from build123d import *

# Parameters (mm, degrees)
F1_DEPTH = 112.7125


with BuildPart() as f1:
    # F0 (on Right) → F1 (new body, symmetric)
    with BuildSketch(Plane.YZ):
        with BuildLine():
            ThreePointArc((-65.019769, 11.612246), (-46.032427, -7.846355), (-24.695704, -24.695704))
            Line((-24.695704, -24.695704), (0, 0))
            Line((0, 0), (0, 34.925))
            ThreePointArc((0, 34.925), (-27.001631, 38.098052), (-54.187018, 37.764821))
            ThreePointArc((-54.187018, 37.764821), (-67.631541, 28.013901), (-65.019769, 11.612246))
        make_face()
    extrude(amount=F1_DEPTH, both=True)


solid = f1.part
The listing builds one solid part. Answer for the finished solid, in the listing's coordinates (mm). Round coordinates to 2 decimals unless told otherwise and drop trailing zeros. Loops run counter-clockwise (first coordinate to the right, second up) from the corner with the lowest first, then second, coordinate; pieces in that order, holes last. Notation, with made-up numbers: M 28,37 L 45,37 A12 cw 45,55 Z; hole C -8,66.5 d3. An arc over 180 degrees is marked long. Write each question's results on one line, items separated by ' | '. Start each with the question number.
1) Find section C-C on y = -12. Write down the section's boundary in (x, z).
2) Find section B-B on z = 28. Write down the section's boundary in (x, y).
3) Each of these flat-tipped pins is pushed along its axis until it touches: pin 1 (6 mm diameter, centred on x = -14, y = -14, fed in from +Z); pin 2 (8 mm diameter, centred on x = 22, y = -7, fed in from -Z); pin 3 (6 mm diameter, centred on x = 43, y = -12, fed in from +Z). Where does it stop, or does it pass through?
4) Find section A-A on x = 78. Write down the section's boundary in (y, z) (3 decimals).
5) Straight lines are drawn through the part: probe 1 along Y at (x, z) = (-83.5, 22.5); probe 2 along Z at (x, y) = (-90, -56); probe 3 along Y at (x, z) = (-39, -2.5). For each, find the intervals that lie inside material, in ascending order.
Final values:
1) outline: M -112.71,-12 L 112.71,-12 L 112.71,36.77 L -112.71,36.77 Z
2) outline: M -112.71,-67.64 L 112.71,-67.64 L 112.71,0 L -112.71,0 Z
3) pin 1: z = 37.33 | pin 2: z = -11 | pin 3: z = 37.12
4) outline: M -65.02,11.612 A210.52 ccw -24.696,-24.696 L 0,0 L 0,34.925 A210.52 ccw -54.187,37.765 A15.872 ccw Z
5) probe 1: -68.83 to 0 | probe 2: 1.74 to 37.52 | probe 3: -51.75 to -2.5
